from build123d import *

# Parameters (mm, degrees)
SKETCH1_R           = 1.6
BOSS_EXTRUDE1_DEPTH = 1.6
SKETCH2_W           = 5
SKETCH2_H           = 7.5
BOSS_EXTRUDE2_DEPTH = 3


with BuildPart() as part:
    # Sketch1 → Boss-Extrude1 (new body)
    with BuildSketch(Plane.XY):
        with BuildLine():
            Line((-13.235657624, 13.611622239), (16.764342376, 13.611622239))
            ThreePointArc((16.764342376, 13.611622239), (18.178555938, 13.025835801), (18.764342376, 11.611622239))
            Line((18.764342376, 11.611622239), (18.764342376, -18.388377761))
            ThreePointArc((18.764342376, -18.388377761), (18.178555938, -19.802591324), (16.764342376, -20.388377761))
            Line((16.764342376, -20.388377761), (-13.235657624, -20.388377761))
            ThreePointArc((-13.235657624, -20.388377761), (-14.649871187, -19.802591324), (-15.235657624, -18.388377761))
            Line((-15.235657624, -18.388377761), (-15.235657624, 11.611622239))
            ThreePointArc((-15.235657624, 11.611622239), (-14.649871187, 13.025835801), (-13.235657624, 13.611622239))
        make_face()
        with Locations((16.764342376, 11.611622239)):
            Circle(SKETCH1_R, mode=Mode.SUBTRACT)
        with Locations(Location((16.764342376, -18.388377761, 0), (0, 0, 180))):
            Circle(SKETCH1_R, mode=Mode.SUBTRACT)
        with Locations(Location((-13.235657624, 11.611622239, 0), (0, 0, 180))):
            Circle(SKETCH1_R, mode=Mode.SUBTRACT)
        with Locations((-13.235657624, -18.388377761)):
            Circle(SKETCH1_R, mode=Mode.SUBTRACT)
    extrude(amount=BOSS_EXTRUDE1_DEPTH)

    # Sketch2 → Boss-Extrude2 (add)
    with BuildSketch(Plane.XY.offset(1.6)):
        with Locations((7.264342376, 2.361622239)):
            Rectangle(SKETCH2_W, SKETCH2_H)
        with Locations((7.264342376, -9.138377761)):
            Rectangle(SKETCH2_W, SKETCH2_H)
        with Locations((-3.735657624, -9.138377761)):
            Rectangle(SKETCH2_W, SKETCH2_H)
        with Locations((-3.735657624, 2.361622239)):
            Rectangle(SKETCH2_W, SKETCH2_H)
    extrude(amount=BOSS_EXTRUDE2_DEPTH)


solid = part.part
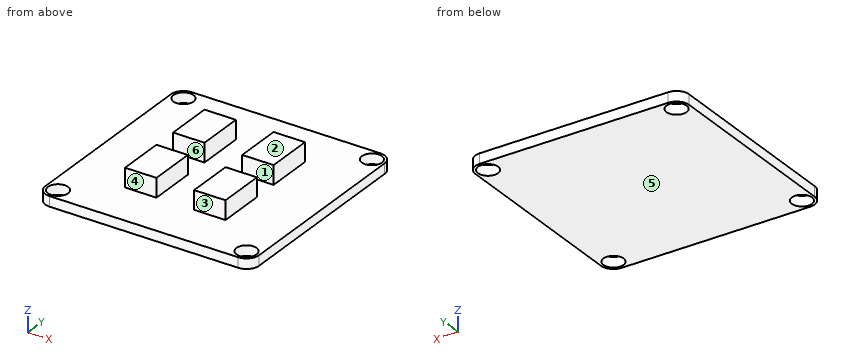
Could you check a few things on this model? Use its own coordinates, in mm. Face numbers are marked on the shaded views. A direction names the side the tool comes from. Round coordinates to 2 decimals unless told otherwise and drop trailing zeros. Loops run counter-clockwise (first coordinate to the right, second up) from the corner with the lowest first, then second, coordinate; pieces in that order, holes last. Notation, with made-up numbers: (56, -4.75) -> (73, -4.75) arc R19 cw to (73, 14.25) -> close; hole circle Ø6 at (-15, 38). An arc over 180 degrees is marked (long way). Use CSV: the item, a comma, the result in double quotes.
(1) Suppose I cut it at B-B on x = -3. Write out the boundary of the cut face in (y, z), plus the area to 3 significant figures.
Return value:
outline,"(-20.39, 0) -> (13.61, 0) -> (13.61, 1.6) -> (6.11, 1.6) -> (6.11, 4.6) -> (-1.39, 4.6) -> (-1.39, 1.6) -> (-5.39, 1.6) -> (-5.39, 4.6) -> (-12.89, 4.6) -> (-12.89, 1.6) -> (-20.39, 1.6) -> close"
area,"99.4 mm²"
(2) Suppose I cut it at C-C on y = -1. Write out the boundary of the cut face in (x, z), plus the area to 3 significant figures.
Return value:
outline,"(-15.24, 0) -> (18.76, 0) -> (18.76, 1.6) -> (9.76, 1.6) -> (9.76, 4.6) -> (4.76, 4.6) -> (4.76, 1.6) -> (-1.24, 1.6) -> (-1.24, 4.6) -> (-6.24, 4.6) -> (-6.24, 1.6) -> (-15.24, 1.6) -> close"
area,"84.4 mm²"
(3) If we mould it in two halves opening along Y, with no side actions, what happens to the marked faces 4, 5 and 6? For each: +Y half, -Y half, draft (parallel to the pull), parting line (faces both ways), or undercut.
Return value:
face 4,"-Y half"
face 5,"draft"
face 6,"undercut"
(4) For the marked faces 1, 2 and 3, which set-ups out of +Z, -Z, +X, -X, +Y, -Y let a thin tool reach every point of the face, with its end or its side?
Return value:
face 1,"+Z, +X, -X"
face 2,"+Z, +X, -X, +Y, -Y"
face 3,"+Z, +X, -X, -Y"
(5) Suppose I cut it at D-D on y = -5. Write out the boundary of the cut face in (x, z), plus the area to 3 significant figures.
Return value:
outline,"(-15.24, 0) -> (18.76, 0) -> (18.76, 1.6) -> (-15.24, 1.6) -> close"
area,"54.4 mm²"
(6) Suppose I cut it at A-A on z = 2.1. Write out the boundary of the cut face in (x, y), plus the area to 3 significant figures.
Return value:
outline,"(-6.24, -12.89) -> (-1.24, -12.89) -> (-1.24, -5.39) -> (-6.24, -5.39) -> close; (-6.24, -1.39) -> (-1.24, -1.39) -> (-1.24, 6.11) -> (-6.24, 6.11) -> close; (4.76, -12.89) -> (9.76, -12.89) -> (9.76, -5.39) -> (4.76, -5.39) -> close; (4.76, -1.39) -> (9.76, -1.39) -> (9.76, 6.11) -> (4.76, 6.11) -> close"
area,"150 mm²"
(7) If I drill on probe 1 along X at (y, z) = (-9.5, 4.35); probe 2 along Y at (x, z) = (8.5, 2.6); probe 3 along Z at (x, y) = (11, -2), over which ranges is the centre line in solid material (lowest first)? Write a range as [from, to].
Return value:
probe 1,"x = [-6.24, -1.24], [4.76, 9.76]"
probe 2,"y = [-12.89, -5.39], [-1.39, 6.11]"
probe 3,"z = [0, 1.6]"
(8) Will these pins go through, and if not, where does the flat tip stop? pin 1 Ø2 at (x, z) = (9, 3.5) entering from +Y; pin 2 Ø1.5 at (y, z) = (1, 2.5) entering from -X; pin 3 Ø0.9 at (y, z) = (3, 2.5) entering from +X; pin 4 Ø1.9 at (x, y) = (-13.24, 11.61) entering from -Z.
Return value:
pin 1,"stops at y = 6.11"
pin 2,"stops at x = -6.24"
pin 3,"stops at x = 9.76"
pin 4,"passes through"
